```python
from build123d import *

# Parameters (mm, degrees)
CUBE013_W                = 3.2
CUBE013_H                = 7.4
CUBE013_DEPTH            = 6
CUBE014_W                = 3.52
CUBE014_H                = 7.4
CUBE014_DEPTH            = 6
CYLINDER009_R            = 2.3
CYLINDER009_DEPTH        = 71
CUBE012_W                = 14
CUBE012_H                = 10
CUBE012_DEPTH            = 6
CYLINDER007_R            = 2.3
CYLINDER007_DEPTH        = 71
CYLINDER008_R            = 2.1
CYLINDER008_DEPTH        = 71
PRISM006_DEPTH           = 57.8
PRISM006_ROLL_ANGLE      = 90
PRISM006_PITCH_ANGLE     = -14.999996
PRISM007_DEPTH           = 57.8
PRISM007_ROLL_ANGLE      = -90
PRISM007_PITCH_ANGLE     = -14.999996
PRISM007_PLACEMENT_ANGLE = -180
PRISM008_DEPTH           = 21
CUBE011_W                = 14
CUBE011_H                = 57.8
CUBE011_DEPTH            = 23
PRISM004_DEPTH           = 20
PRISM004_ROLL_ANGLE      = 90
PRISM004_PITCH_ANGLE     = -14.999988
PRISM004_PLACEMENT_ANGLE = 90
PRISM005_DEPTH           = 20
PRISM005_ROLL_ANGLE      = -90
PRISM005_PITCH_ANGLE     = -14.999988
PRISM005_PLACEMENT_ANGLE = -90
CUBE010_W                = 20
CUBE010_H                = 63.8
CUBE010_DEPTH            = 23


with BuildPart() as cube013:
    # cube013 → cube013 (new body)
    with BuildSketch(Plane(origin=(-7, -3.7, 8.5), x_dir=(1, 0, 0), z_dir=(0, 0, 1))):
        with Locations((1.6, 3.7)):
            Rectangle(CUBE013_W, CUBE013_H)
    extrude(amount=CUBE013_DEPTH)


with BuildPart() as cube014:
    # cube014 → cube014 (new body)
    with BuildSketch(Plane(origin=(2.85194, -3.7, 8.5), x_dir=(1, 0, 0), z_dir=(0, 0, 1))):
        with Locations((1.76, 3.7)):
            Rectangle(CUBE014_W, CUBE014_H)
    extrude(amount=CUBE014_DEPTH)


with BuildPart() as group005:
    # cylinder009 → cylinder009 (new body)
    with BuildSketch(Plane(origin=(-35.5, 0, 11.75), x_dir=(0, 1, 0), z_dir=(1, 0, 0))):
        Circle(CYLINDER009_R)
    extrude(amount=CYLINDER009_DEPTH)

    # Group005: union cube013, cube014
    add(cube013.part)
    add(cube014.part)


with BuildPart() as body003:
    # cube012 → cube012 (new body)
    with BuildSketch(Plane(origin=(-7, -5, 8.5), x_dir=(1, 0, 0), z_dir=(0, 0, 1))):
        with Locations((7, 5)):
            Rectangle(CUBE012_W, CUBE012_H)
    extrude(amount=CUBE012_DEPTH)

    # difference003: cut Group005
    add(group005.part, mode=Mode.SUBTRACT)


with BuildPart() as cylinder007:
    # cylinder007 → cylinder007 (new body)
    with BuildSketch(Plane(origin=(-35.5, 0, 11.75), x_dir=(0, 1, 0), z_dir=(1, 0, 0))):
        Circle(CYLINDER007_R)
    extrude(amount=CYLINDER007_DEPTH)


with BuildPart() as cylinder008:
    # cylinder008 → cylinder008 (new body)
    with BuildSketch(Plane(origin=(0, 35.5, 25.75), x_dir=(1, 0, 0), z_dir=(0, -1, 0))):
        Circle(CYLINDER008_R)
    extrude(amount=CYLINDER008_DEPTH)


with BuildPart() as prism006:
    # prism006 → prism006 (new body)
    with BuildSketch(Plane.XY):
        Polygon((3, 0), (-1.5, 2.598076), (-1.5, -2.598076), align=None)
    extrude(amount=PRISM006_DEPTH)


with BuildPart() as prism006_1:
    # prism006 roll: moved
    add(prism006.part.rotate(Axis((0, 0, 0), (1, 0, 0)), PRISM006_ROLL_ANGLE))


with BuildPart() as prism006_2:
    # prism006 pitch: moved
    add(prism006_1.part.rotate(Axis((0, 0, 0), (0, 1, 0)), PRISM006_PITCH_ANGLE))


with BuildPart() as prism006_3:
    # prism006 placement: moved
    add(prism006_2.part.moved(Location((7, 28.900002, 31.5))))


with BuildPart() as prism007:
    # prism007 → prism007 (new body)
    with BuildSketch(Plane.XY):
        Polygon((3, 0), (-1.5, 2.598076), (-1.5, -2.598076), align=None)
    extrude(amount=PRISM007_DEPTH)


with BuildPart() as prism007_1:
    # prism007 roll: moved
    add(prism007.part.rotate(Axis((0, 0, 0), (1, 0, 0)), PRISM007_ROLL_ANGLE))


with BuildPart() as prism007_2:
    # prism007 pitch: moved
    add(prism007_1.part.rotate(Axis((0, 0, 0), (0, 1, 0)), PRISM007_PITCH_ANGLE))


with BuildPart() as prism007_3:
    # prism007 placement: moved
    add(prism007_2.part.moved(Location((-7, 28.900002, 31.5))).rotate(Axis((-7, 28.900002, 31.5), (0, 0, 1)), PRISM007_PLACEMENT_ANGLE))


with BuildPart() as prism008:
    # prism008 → prism008 (new body)
    with BuildSketch(Plane(origin=(-10.5, -21.9, 25.75), x_dir=(0, 1, 0), z_dir=(1, 0, 0))):
        Polygon((3.1, 0), (1.55, 2.684679), (-1.55, 2.684679), (-3.1, 0), (-1.55, -2.684679), (1.55, -2.684679), align=None)
    extrude(amount=PRISM008_DEPTH)


with BuildPart() as group004:
    # cube011 → cube011 (new body)
    with BuildSketch(Plane(origin=(-7, -28.9, 8.5), x_dir=(1, 0, 0), z_dir=(0, 0, 1))):
        with Locations((7, 28.9)):
            Rectangle(CUBE011_W, CUBE011_H)
    extrude(amount=CUBE011_DEPTH)

    # Group004: union cylinder007, cylinder008, prism006, prism007, prism008
    add(cylinder007.part)
    add(cylinder008.part)
    add(prism006_3.part)
    add(prism007_3.part)
    add(prism008.part)


with BuildPart() as prism004:
    # prism004 → prism004 (new body)
    with BuildSketch(Plane.XY):
        Polygon((3, 0), (-1.5, 2.598076), (-1.5, -2.598076), align=None)
    extrude(amount=PRISM004_DEPTH)


with BuildPart() as prism004_1:
    # prism004 roll: moved
    add(prism004.part.rotate(Axis((0, 0, 0), (1, 0, 0)), PRISM004_ROLL_ANGLE))


with BuildPart() as prism004_2:
    # prism004 pitch: moved
    add(prism004_1.part.rotate(Axis((0, 0, 0), (0, 1, 0)), PRISM004_PITCH_ANGLE))


with BuildPart() as prism004_3:
    # prism004 placement: moved
    add(prism004_2.part.moved(Location((-10.000001, 32, 16.6))).rotate(Axis((-10.000001, 32, 16.6), (0, 0, 1)), PRISM004_PLACEMENT_ANGLE))


with BuildPart() as prism005:
    # prism005 → prism005 (new body)
    with BuildSketch(Plane.XY):
        Polygon((3, 0), (-1.5, 2.598076), (-1.5, -2.598076), align=None)
    extrude(amount=PRISM005_DEPTH)


with BuildPart() as prism005_1:
    # prism005 roll: moved
    add(prism005.part.rotate(Axis((0, 0, 0), (1, 0, 0)), PRISM005_ROLL_ANGLE))


with BuildPart() as prism005_2:
    # prism005 pitch: moved
    add(prism005_1.part.rotate(Axis((0, 0, 0), (0, 1, 0)), PRISM005_PITCH_ANGLE))


with BuildPart() as prism005_3:
    # prism005 placement: moved
    add(prism005_2.part.moved(Location((-10.000001, -32, 16.6))).rotate(Axis((-10.000001, -32, 16.6), (0, 0, 1)), PRISM005_PLACEMENT_ANGLE))


with BuildPart() as bottom_slider:
    # cube010 → cube010 (new body)
    with BuildSketch(Plane(origin=(-10, -31.9, 8.5), x_dir=(1, 0, 0), z_dir=(0, 0, 1))):
        with Locations((10, 31.9)):
            Rectangle(CUBE010_W, CUBE010_H)
    extrude(amount=CUBE010_DEPTH)

    # Group003: union prism004, prism005
    add(prism004_3.part)
    add(prism005_3.part)

    # difference002: cut Group004
    add(group004.part, mode=Mode.SUBTRACT)

    # Fusion: union Body003
    add(body003.part)


solid = bottom_slider.part
```
Design review of the part built by this model. Coordinates are the model's own, in mm. A direction names the side the tool comes from. Coordinates: 2 decimals unless noted, no trailing zeros. Loops run counter-clockwise (first coordinate to the right, second up) from the corner with the lowest first, then second, coordinate; pieces in that order, holes last. Notation, with made-up numbers: (9.5, 64) -> (62.5, 64) arc R26 cw to (62.5, 84) -> close; hole circle Ø3 at (27, 58.5). An arc over 180 degrees is marked (long way). Answer as a JSON object with one key per item and string values.
Q1. Take a section at D-D on z = 22.25. Give the boundary of the cut face in (x, y).
Answer block:
{"outline": "(-10, -31.9) -> (10, -31.9) -> (10, 31.9) -> (-10, 31.9) -> close; hole (-7, -28.9) -> (7, -28.9) -> (7, 28.9) -> (-7, 28.9) -> close"}
Q2. The part is to be moulded in two halves that separate along Z. For faces 4 (the flat face through (0, 31.9, 20)), 5 (the flat face through (-0.14, -33.49, 15.97)), 6 (the flat face through (8.48, -19.56, 27.07)), 7 (the flat face through (-8.521, -24.214, 27.111)), say which applies: +Z half, -Z half, draft (parallel to the pull), parting line (faces both ways), or undercut.
Answer block:
{"face 4": "draft", "face 5": "-Z half", "face 6": "undercut", "face 7": "undercut"}
Q3. Take a section at A-A on z = 11.75. Give the number of separate pieces and of enclosed holes in the cut face, plus the area to 3 significant figures.
Answer block:
{"separate pieces": "2", "enclosed holes": "2", "area": "496 mm^2"}
Q4. Take a section at B-B on x = 0. Give the boundary of the cut face in (y, z).
Answer block:
{"outline": "(-34.9, 17.38) -> (-31.9, 14.38) -> (-31.9, 8.5) -> (-28.9, 8.5) -> (-28.9, 23.65) -> (-31.9, 23.65) -> (-31.9, 18.18) -> close; (-31.9, 27.85) -> (-28.9, 27.85) -> (-28.9, 31.5) -> (-31.9, 31.5) -> close; (-5, 8.5) -> (5, 8.5) -> (5, 14.5) -> (-5, 14.5) -> close; (28.9, 8.5) -> (31.9, 8.5) -> (31.9, 14.38) -> (34.9, 17.38) -> (31.9, 18.18) -> (31.9, 23.65) -> (28.9, 23.65) -> close; (28.9, 27.85) -> (31.9, 27.85) -> (31.9, 31.5) -> (28.9, 31.5) -> close; hole circle Ø4.6 at (0, 11.75)"}
Q5. Take a section at C-C on y = 0. Give the boundary of the cut face in (x, z).
Answer block:
{"outline": "(-10, 8.5) -> (-7, 8.5) -> (-7, 9.45) -> (-10, 9.45) -> close; (-10, 14.05) -> (-7, 14.05) -> (-7, 29.38) -> (-9.12, 31.5) -> (-10, 31.5) -> close; (-3.8, 8.5) -> (2.85, 8.5) -> (2.85, 9.45) -> (-3.8, 9.45) -> close; (-3.8, 14.05) -> (2.85, 14.05) -> (2.85, 14.5) -> (-3.8, 14.5) -> close; (6.37, 8.5) -> (10, 8.5) -> (10, 9.45) -> (6.37, 9.45) -> close; (6.37, 14.05) -> (10, 14.05) -> (10, 31.5) -> (9.12, 31.5) -> (7, 29.38) -> (7, 14.5) -> (6.37, 14.5) -> close"}
Q6. Tool access review of faces 1 (the flat face through (-9.7, 0.1, 31.5)), 2 (the flat face through (8, -22, 23.065)), 3 (the flat face through (5, 3.7, 11)): name each direction out of +Z, -Z, +X, -X, +Y, -Y from which nothing blocks a thin tool from reaching the whole face with its end or side.
Answer block:
{"face 1": "+Z, +X, -X, +Y, -Y", "face 2": "+X, -X", "face 3": "+Z, -Z"}
Q7. Clearance check with flat-ended pins moving along their axes: pin 1 Ø2.5 at (x, z) = (-5.5, 10) entering from +Y; pin 2 Ø6 at (x, z) = (2, 22) entering from -Y; pin 3 Ø1.8 at (y, z) = (-0.5, 12.5) entering from -X; pin 4 Ø11 at (x, z) = (2.5, 17.5) entering from -Y. State where each tip first meets the part, or that it passes through.
Answer block:
{"pin 1": "stops at y = 31.9", "pin 2": "stops at y = -31.9", "pin 3": "passes through", "pin 4": "stops at y = -34.9"}
Q8. To check wall thickness, follow L1, parallel to Y at x = -1, z = 11.75; L2, parallel to X at y = 30.45, z = 25.75; L3, parallel to Y at x = -0.25, z = 23.25. State the ranges of each line that lie inside material, in increasing order.
Answer block:
{"L1": "y = -31.9 to -28.9, -5 to -2.3, 2.3 to 5, 28.9 to 31.9", "L2": "x = -10 to -2.1, 2.1 to 10", "L3": "y = -31.9 to -28.9, 28.9 to 31.9"}
